Source: CAD feature listing. Evaluate the final solid. Frame: model axes, mm. Coordinates: 2 decimals unless noted, no trailing zeros. One line per item, written item: value. Start each with the question number.
1. Mould query, pull axis Z, two halves, no side actions, for faces 1 (the flat face through (15, 0, 0)), 2 (the flat face through (0, 0, 11)). Classes: released by +Z, released by -Z, zero draft, split by the parting line, or undercut.
2. First-contact query: P1, Ø5, axis at x = 4, y = 4, coming from the +Z side; P2, Ø1.5, axis at x = 18.5, y = -3, coming from the -Z side; P3, Ø12, axis at x = 14, y = 9, coming from the +Z side. Flat tips, straight axial feed; report the tip coordinate or a pass-through.
3. Line query: line 1 (X direction, y = 11, z = -0.5); line 2 (X direction, y = -10.5, z = -4). Output: solid intervals per line, ascending.
from build123d import *

# Parameters (mm, degrees)
SKETCH2_R           = 25
BOSS_EXTRUDE1_DEPTH = 25
FILLET1_R           = 25
SKETCH3_R           = 13
CUT_EXTRUDE1_DEPTH  = 15
THREAD2_PITCH       = 5
SKETCH17_W          = 32.265191549
SKETCH17_H          = 31.135556834
CUT_EXTRUDE2_DEPTH  = 70


with BuildPart() as part:
    # Sketch2 → Boss-Extrude1 (new body)
    with BuildSketch(Plane(origin=(0, 0, 0), x_dir=(0, 0, -1), z_dir=(1, 0, 0))):
        Circle(SKETCH2_R)
    extrude(amount=BOSS_EXTRUDE1_DEPTH)

    # Fillet1
    fillet1_edges = [part.edges().sort_by_distance(p)[0] for p in [
        (25, 0, 25),
    ]]
    fillet(fillet1_edges, radius=FILLET1_R - 0.0001)  # a hair under: the kernel refuses the full size

    # Sketch3 → Cut-Extrude1 (cut)
    with BuildSketch(Plane.ZY):
        Circle(SKETCH3_R)
    extrude(amount=-CUT_EXTRUDE1_DEPTH, mode=Mode.SUBTRACT)

    # Thread2: the profile of Thread Profile3 profile screwed along a right-hand helix of 3 turns, 12 arcs to a turn; built about Z, then put on its axis
    thread2_z = Axis((0, 0, 0), (0, 0, 1))
    thread2_corners = [(13.0003, -3e-09, -0.000173205), (13.0003, -3e-09, 4.375173191), (10.293670625, -3e-09, 2.812499993), (10.293670625, -3e-09, 1.562499993)]
    with BuildLine(mode=Mode.PRIVATE) as thread2_profile:
        Line(thread2_corners[0], thread2_corners[1])
        Line(thread2_corners[1], thread2_corners[2])
        Line(thread2_corners[2], thread2_corners[3])
        Line(thread2_corners[3], thread2_corners[0])
    thread2_cap = Face(thread2_profile.wire())
    thread2_turn_angles = [0, 15, 30, 45, 60, 75, 90, 105, 120, 135, 150, 165, 180, 195, 210, 225, 240, 255, 270, 285, 300, 315, 330, 345, 360]
    thread2_turn_weights = [1, 0.9659258262890683, 1, 0.9659258262890683, 1, 0.9659258262890683, 1, 0.9659258262890683, 1, 0.9659258262890683, 1, 0.9659258262890683, 1, 0.9659258262890683, 1, 0.9659258262890683, 1, 0.9659258262890683, 1, 0.9659258262890683, 1, 0.9659258262890683, 1, 0.9659258262890683, 1]
    thread2_turn_rails = [Edge.make_bspline([Vector(p[0], p[1], 0).rotate(thread2_z, thread2_turn_angles[k]) / thread2_turn_weights[k] + Vector(0, 0, p[2] + THREAD2_PITCH * thread2_turn_angles[k] / 360) for k in range(25)], [0, 0, 0, 1, 1, 2, 2, 3, 3, 4, 4, 5, 5, 6, 6, 7, 7, 8, 8, 9, 9, 10, 10, 11, 11, 12, 12, 12], 2, thread2_turn_weights) for p in thread2_corners]
    thread2_turn_sides = [Face.make_surface_from_curves(thread2_turn_rails[p[0]], thread2_turn_rails[p[1]]) for p in [(0, 1), (1, 2), (2, 3), (3, 0)]]
    thread2 = Plane(origin=(-4, 0, 0), x_dir=(0, 0.087155743, -0.996194698), z_dir=(1, 0, 0)) * Solid(Shell([*[p.moved(Location((0, 0, THREAD2_PITCH * i))) for i in range(3) for p in thread2_turn_sides], thread2_cap, thread2_cap.rotate(thread2_z, 1080).moved(Location((0, 0, THREAD2_PITCH * 1080 / 360)))]))
    add(thread2)

    # Sketch17 → Cut-Extrude2 (cut)
    with BuildSketch(Plane.ZY):
        with Locations((0.529516272, -0.282408679)):
            Rectangle(SKETCH17_W, SKETCH17_H)
    extrude(amount=CUT_EXTRUDE2_DEPTH, mode=Mode.SUBTRACT)


solid = part.part
Computed values:
1. face 1: undercut
1. face 2: zero draft
2. P1: stops at z = 24.8
2. P2: stops at z = -17.36
2. P3: stops at z = 22.62
3. line 1: x = 0 to 0.37, 3.29 to 5.37, 8.29 to 10.37, 15 to 22.44
3. line 2: x = 0.99 to 3.33, 5.99 to 8.33, 10.99 to 13.33, 15 to 22.33
